Read the model definition and answer for the solid it produces. Units are mm, in the model's axes. A direction names the side the tool comes from. Give positions to 0.01 mm unless a question says otherwise; leave off trailing zeros. Write each loop counter-clockwise with the first axis right and the second up, starting at its lowest first coordinate (ties: lowest second). Pieces come first, ordered by that corner, then holes. Notation, with made-up numbers: (52.5, -33.5) -> (79.5, -33.5) arc R24 ccw to (79.5, -20.5) -> close; hole circle Ø5 at (-17.75, 1). An arc over 180 degrees is marked (long way). Use a Markdown table: item, result.
from build123d import *

# Parameters (mm, degrees)
BASPROSKE_W         = 7
BASPROSKE_H         = 6.86
TOOTHCUT_DEPTH      = 12.963243707
TEETHCUTS_COUNT     = 12
TEETHCUTS_ANGLE     = 330
BORSKE_R            = 1
BORE_DEPTH          = 50.0000508
SKETCH1_R           = 12.5
BOSS_EXTRUDE1_DEPTH = 12
SKETCH2_R           = 1.65
CUT_EXTRUDE1_DEPTH  = 22.365860619
SKETCH3_R           = 3
CUT_EXTRUDE2_DEPTH  = 9
CIRPATTERN1_COUNT   = 4
CHAMFER1_SIZE       = 4
SKETCH4_R           = 2.25
CUT_EXTRUDE3_DEPTH  = 6


with BuildPart() as part:
    # BasProSke → Base-Revolve (revolve)
    with BuildSketch(Plane(origin=(0, 0, 0), x_dir=(1, 0, 0), z_dir=(0, 1, 0)), mode=Mode.PRIVATE) as base_revolve_sk:
        with Locations((3.5, 3.43)):
            Rectangle(BASPROSKE_W, BASPROSKE_H)
    revolve(base_revolve_sk.sketch.rotate(Axis((-10, 0, 0), (1, 0, 0)), 180), axis=Axis((-10, 0, 0), (1, 0, 0)))

    # TooCutSke → ToothCut (cut, through all)
    with BuildSketch(Plane(origin=(0, 0, 0), x_dir=(0, 0, -1), z_dir=(1, 0, 0))):
        with BuildLine():
            ThreePointArc((0.552016647, 4.621146354), (0, 4.654), (-0.552016647, 4.621146354))
            ThreePointArc((-0.552016647, 4.621146354), (-0.822258441, 5.798784691), (-1.641510828, 6.686865885))
            ThreePointArc((-1.641510828, 6.686865885), (0, 6.8854), (1.641510828, 6.686865885))
            ThreePointArc((1.641510828, 6.686865885), (0.822258441, 5.798784691), (0.552016647, 4.621146354))
        make_face()
    toothcut = extrude(amount=TOOTHCUT_DEPTH, mode=Mode.SUBTRACT)

    # TeethCuts: ToothCut ×12 about axis
    teethcuts_axis = Axis((-10, 0, 0), (1, 0, 0))
    for i in range(1, TEETHCUTS_COUNT):
        add(toothcut.rotate(teethcuts_axis, i * TEETHCUTS_ANGLE / (TEETHCUTS_COUNT - 1)), mode=Mode.SUBTRACT)

    # BorSke → Bore (cut, symmetric)
    with BuildSketch(Plane(origin=(0, 0, 0), x_dir=(0, 0, -1), z_dir=(1, 0, 0))):
        with Locations(Location((0, 0, 0), (0, 0, 180))):
            Circle(BORSKE_R)
    extrude(amount=BORE_DEPTH, both=True, mode=Mode.SUBTRACT)

    # Sketch1 → Boss-Extrude1 (add)
    with BuildSketch(Plane(origin=(7, 0, 0), x_dir=(0, 0, -1), z_dir=(1, 0, 0))):
        Circle(SKETCH1_R)
    extrude(amount=BOSS_EXTRUDE1_DEPTH)

    # Sketch2 → Cut-Extrude1 (cut, through all)
    with BuildSketch(Plane.ZY.offset(-7)):
        with Locations((0, 9)):
            Circle(SKETCH2_R)
    cut_extrude1 = extrude(amount=-CUT_EXTRUDE1_DEPTH, mode=Mode.SUBTRACT)

    # Sketch3 → Cut-Extrude2 (cut)
    with BuildSketch(Plane.ZY.offset(-7)):
        with Locations(Location((0, 9, 0), (0, 0, 307.326549715))):
            Circle(SKETCH3_R)
    cut_extrude2 = extrude(amount=-CUT_EXTRUDE2_DEPTH, mode=Mode.SUBTRACT)

    # CirPattern1: Cut-Extrude1, Cut-Extrude2 ×4 about axis
    cirpattern1_axis = Axis((0, 0, 0), (1, 0, 0))
    add([cut_extrude1.rotate(cirpattern1_axis, i * 360 / CIRPATTERN1_COUNT) for i in range(1, CIRPATTERN1_COUNT)], mode=Mode.SUBTRACT)
    add([cut_extrude2.rotate(cirpattern1_axis, i * 360 / CIRPATTERN1_COUNT) for i in range(1, CIRPATTERN1_COUNT)], mode=Mode.SUBTRACT)

    # Chamfer1
    # the kernel refuses this chamfer: 4 mm, written as the material it takes off along each edge
    with BuildSketch(Plane(origin=(7, 0, 0), x_dir=(0, 0, -1), z_dir=(0, -1, 0))) as chamfer1_piece_1:
        Polygon((12.5, CHAMFER1_SIZE), (12.5 - CHAMFER1_SIZE, 0), (12.5, 0), align=None)
    revolve(axis=Axis((7, 0, 0), (1, 0, 0)), mode=Mode.SUBTRACT)

    # Sketch4 → Cut-Extrude3 (cut)
    with BuildSketch(Plane(origin=(19, 0, 0), x_dir=(0, 0, -1), z_dir=(1, 0, 0))):
        Circle(SKETCH4_R)
    extrude(amount=-CUT_EXTRUDE3_DEPTH, mode=Mode.SUBTRACT)


solid = part.part
Item 1: Straight lines are drawn through the part: line 1 along Y through (x, z) = (14, 1.5); line 2 along Y through (x, z) = (12.5, 2.5); line 3 along Z through (x, y) = (5, -4.25). For each, find the intervals that lie inside material, in ascending order. Write a range as [from, to].
Return value:
| item | result |
|---|---|
| line 1 | [-12.41, -11.6], [-6.4, -1.68], [1.68, 6.4], [11.6, 12.41] |
| line 2 | [-12.25, -10.66], [-7.34, 7.34], [10.66, 12.25] |
| line 3 | [-4.89, -3.17], [-1.9, 1.9], [3.17, 4.89] |
Item 2: A tool of negligible diameter and unlimited length cuts with its end or side. For faces 1 (the face through (7, -5, 0)), 2 (the face through (16.04, 2.23, 0.29)), 3 (the face through (7, 0, 0)), from which of +Z, -Z, +X, -X, +Y, -Y can it reach the whole face along a straight path? Write none if from no direction.
Return value:
| item | result |
|---|---|
| face 1 | -X, -Y |
| face 2 | +X |
| face 3 | -X |
Item 3: Each of these flat-tipped pins is pushed along its axis until it touches: P1, Ø5, axis at y = -0.5, z = 8, coming from the -X side; P2, Ø2, axis at y = -7.5, z = 8.5, coming from the -X side; P3, Ø8, axis at x = 6.5, z = 5.5, coming from the +Y side; P4, Ø5, axis at x = 2.5, z = 0, coming from the -Y side. Where does it stop, or does it pass through?
Return value:
| item | result |
|---|---|
| P1 | x = 0 |
| P2 | x = 8.84 |
| P3 | y = 11.01 |
| P4 | y = -6.67 |
Item 4: A cutting plane is placed at C-C (x = 12). Give the vertices of the cut face in (y, z), then the cut area to 3 significant figures.
Return value:
| item | result |
|---|---|
| outline | circle Ø25 at (0, 0); hole circle Ø6 at (-9, 0); hole circle Ø6 at (0, -9); hole circle Ø6 at (0, 9); hole circle Ø6 at (9, 0) |
| area | 378 mm^2 |
Item 5: A cutting plane is placed at A-A (y = 0). Count the separate pieces of the cut face and the enclosed holes in it, then the cut area to 3 significant figures.
Return value:
| item | result |
|---|---|
| separate pieces | 3 |
| enclosed holes | 0 |
| area | 193 mm^2 |
